Geometry check sheet. Reference: the model listing, model coordinates, mm. Face numbers are marked on the shaded views. A direction names the side the tool comes from. Round coordinates to 2 decimals unless told otherwise and drop trailing zeros. Write each loop counter-clockwise with the first axis right and the second up, starting at its lowest first coordinate (ties: lowest second). Pieces come first, ordered by that corner, then holes. Notation, with made-up numbers: M 10.25,32.5 L 18.25,32.5 A23 cw 18.25,44.5 Z; hole C -39.5,60 d11. An arc over 180 degrees is marked long. Use a Markdown table: item, result.
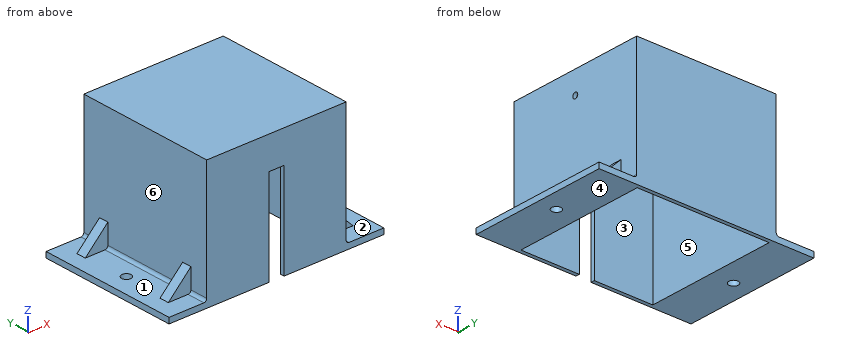
```python
from build123d import *

# Parameters (mm, degrees)
SKETCH_1_W          = 74
SKETCH_1_H          = 74
SKETCH_1_W_2        = 70
SKETCH_1_H_2        = 70
EXTRUDE_1_DEPTH     = 65
SKETCH_2_W          = 74
SKETCH_2_H          = 74
EXTRUDE_2_DEPTH     = 2
SKETCH_3_W          = 20
SKETCH_3_H          = 74
EXTRUDE_3_DEPTH     = 3
EXTRUDE_4_DEPTH     = 2.5
EXTRUDE_5_DEPTH     = 2.5
SKETCH_6_R          = 2.5
CUT_EXTRUDE_1_DEPTH = 5
FILLET_1_R          = 1.5
SKETCH_7_W          = 8
SKETCH_7_H          = 50
CUT_EXTRUDE_2_DEPTH = 5
SKETCH_9_R          = 1.5
CUT_EXTRUDE_3_DEPTH = 5


with BuildPart() as part:
    # 草图1 → 凸台-拉伸1 (new body)
    with BuildSketch(Plane.XY):
        Rectangle(SKETCH_1_W, SKETCH_1_H)
        Rectangle(SKETCH_1_W_2, SKETCH_1_H_2, mode=Mode.SUBTRACT)
    extrude(amount=EXTRUDE_1_DEPTH)

    # 草图2 → 凸台-拉伸2 (add)
    with BuildSketch(Plane.XY.offset(65)):
        Rectangle(SKETCH_2_W, SKETCH_2_H)
    extrude(amount=EXTRUDE_2_DEPTH)

    # 草图3 → 凸台-拉伸3 (add)
    with BuildSketch(Plane(origin=(0, 0, 0), x_dir=(-1, 0, 0), z_dir=(0, 0, -1))):
        with Locations((-47, 0)):
            Rectangle(SKETCH_3_W, SKETCH_3_H)
        with Locations((47, 0)):
            Rectangle(SKETCH_3_W, SKETCH_3_H)
    extrude(amount=-EXTRUDE_3_DEPTH)

    # 草图4 → 凸台-拉伸4 (add, symmetric)
    with BuildSketch(Plane(origin=(0, 25, 0), x_dir=(1, 0, 0), z_dir=(0, 1, 0))):
        Polygon((-37, -15), (-49, -3), (-37, -3), align=None)
    extrude_4 = extrude(amount=EXTRUDE_4_DEPTH, both=True)

    # 草图5 → 凸台-拉伸5 (add, symmetric)
    with BuildSketch(Plane(origin=(0, -25, 0), x_dir=(1, 0, 0), z_dir=(0, 1, 0))):
        Polygon((-37, -15), (-37, -3), (-49, -3), align=None)
    extrude_5 = extrude(amount=EXTRUDE_5_DEPTH, both=True)

    # 镜向1: 凸台-拉伸4, 凸台-拉伸5 across plane
    add(extrude_4.mirror(Plane(origin=(0, 0, 0), x_dir=(0, 0, 1), z_dir=(1, 0, 0))))
    add(extrude_5.mirror(Plane(origin=(0, 0, 0), x_dir=(0, 0, 1), z_dir=(1, 0, 0))))

    # 草图6 → 切除-拉伸1 (cut)
    with BuildSketch(Plane.XY.offset(3)):
        with Locations((47, 0)):
            Circle(SKETCH_6_R)
        with Locations((-47, 0)):
            Circle(SKETCH_6_R)
    extrude(amount=-CUT_EXTRUDE_1_DEPTH, mode=Mode.SUBTRACT)

    # 圆角1
    fillet_1_edges = [part.edges().sort_by_distance(p)[0] for p in [
        (37, 0, 3),
        (-37, 32.25, 3),
        (37, -32.25, 3),
        (-37, 0, 3),
        (-37, -32.25, 3),
        (37, 32.25, 3),
    ]]
    fillet(fillet_1_edges, radius=FILLET_1_R)

    # 草图7 → 切除-拉伸2 (cut)
    with BuildSketch(Plane.XZ.offset(37)):
        with Locations((0, 25)):
            Rectangle(SKETCH_7_W, SKETCH_7_H)
    extrude(amount=-CUT_EXTRUDE_2_DEPTH, mode=Mode.SUBTRACT)

    # 草图9 → 切除-拉伸3 (cut)
    with BuildSketch(Plane(origin=(37, 0, 0), x_dir=(0, 0, -1), z_dir=(1, 0, 0))):
        with Locations((-55, 0)):
            Circle(SKETCH_9_R)
    extrude(amount=-CUT_EXTRUDE_3_DEPTH, mode=Mode.SUBTRACT)


solid = part.part
```
Item 1: Cross-section at C-C, the plane x = -47. Record the cut outline in (y, z), and give its area (3 significant figures).
Outcome:
| item | result |
|---|---|
| outline | M -37,0 L -2.5,0 L -2.5,3 L -22.5,3 L -22.5,5 L -27.5,5 L -27.5,3 L -37,3 Z; M 2.5,0 L 37,0 L 37,3 L 27.5,3 L 27.5,5 L 22.5,5 L 22.5,3 L 2.5,3 Z |
| area | 227 mm2 |
Item 2: Material ranges on line 1 along Y through (x, z) = (34.5, 9); line 2 along Y through (x, z) = (36.65, 55), recorded low to high. Write a range as from..to.
Outcome:
| item | result |
|---|---|
| line 1 | y = -37..-35, 35..37 |
| line 2 | y = -37..-1.5, 1.5..37 |
Item 3: Cross-section at A-A, the plane z = 62. Record the cut outline in (x, y), and give its area (3 significant figures).
Outcome:
| item | result |
|---|---|
| outline | M -37,-37 L 37,-37 L 37,37 L -37,37 Z; hole M -35,-35 L 35,-35 L 35,35 L -35,35 Z |
| area | 576 mm2 |
Item 4: Go/stop test with flat-tipped pins: pin 1 (19.5 mm diameter, centred on y = -1, z = 34.5, fed in from -X); pin 2 (9 mm diameter, centred on x = -48.5, y = 2, fed in from +Z); pin 3 (1.5 mm diameter, centred on x = -3, z = 38.5, fed in from -Y); pin 4 (3 mm diameter, centred on x = 47, y = 0, fed in from -Z). Record where each tip stops, or that it passes through.
Outcome:
| item | result |
|---|---|
| pin 1 | stops at x = -37 |
| pin 2 | stops at z = 3 |
| pin 3 | stops at y = 35 |
| pin 4 | passes through |
Item 5: Cross-section at B-B, the plane y = 0. Record the cut outline in (x, z).
Outcome:
| item | result |
|---|---|
| outline | M -57,0 L -49.5,0 L -49.5,3 L -57,3 Z; M -44.5,0 L -35,0 L -35,65 L 35,65 L 35,56.5 L 37,56.5 L 37,67 L -37,67 L -37,4.5 A1.5 cw -38.5,3 L -44.5,3 Z; M 35,0 L 44.5,0 L 44.5,3 L 38.5,3 A1.5 cw 37,4.5 L 37,53.5 L 35,53.5 Z; M 49.5,0 L 57,0 L 57,3 L 49.5,3 Z |
Item 6: Cross-section at D-D, the plane x = 6. Record the cut outline in (y, z), and give its area (3 significant figures).
Outcome:
| item | result |
|---|---|
| outline | M -37,0 L -35,0 L -35,65 L 35,65 L 35,0 L 37,0 L 37,67 L -37,67 Z |
| area | 408 mm2 |
Item 7: Mould release check, pull along X, two halves, no side actions. Record for the marked faces 4, 5 and 6: +X half, -X half, draft (parallel to the pull), parting line (faces both ways), or undercut.
Outcome:
| item | result |
|---|---|
| face 4 | draft |
| face 5 | undercut |
| face 6 | -X half |
Item 8: Access from +Z, -Z, +X, -X, +Y, -Y to the whole of each face (thin tool, end or side, straight path). Record for the marked faces 1, 2 and 3.
Outcome:
| item | result |
|---|---|
| face 1 | +Z, -X |
| face 2 | +Z, +X |
| face 3 | -Z |
